Autodesk Inventor part; units mm, degrees
ref_plane "YZ Plane" through (0, 0, 0) normal (1, 0, 0) x (0, 1, 0)
ref_plane "XZ Plane" through (0, 0, 0) normal (0, 1, 0) x (-1, 0, 0)
ref_plane "XY Plane" through (0, 0, 0) normal (0, 0, 1) x (1, 0, 0)
sketch "Sketch1" plane through (0, 0, 0) normal (0, 0, 1) x (1, 0, 0)
  circle A0 centre (0, 0) radius 83.82
  dimension "d0" = 167.64
extrude "Extrusion1" add sketch "Sketch1" along normal mid plane 5.08
sketch "Sketch2" plane through (0, 0, 2.54) normal (0, 0, 1) x (1, 0, 0)
  circle A0 centre (0, 80.01) radius 1.7526
  circle A1 centre (-56.5756, 56.5756) radius 1.7526
  circle A2 centre (-80.01, 0) radius 1.7526
  circle A3 centre (-56.5756, -56.5756) radius 1.7526
  circle A4 centre (0, -80.01) radius 1.7526
  circle A5 centre (56.5756, -56.5756) radius 1.7526
  circle A6 centre (80.01, 0) radius 1.7526
  circle A7 centre (56.5756, 56.5756) radius 1.7526
  point P0 (0, 0)
  dimension "d3" = 3.5052
  dimension "d6" = 360
extrude "Extrusion2" cut sketch "Sketch2" against normal through all
sketch "Sketch3" plane through (0, 0, 2.54) normal (0, 0, 1) x (1, 0, 0)
  circle A0 centre (0, 40.9092) radius 1.7526
  circle A1 centre (-28.9272, 28.9272) radius 1.7526
  circle A2 centre (28.9272, 28.9272) radius 1.7526
  circle A3 centre (-40.9092, 0) radius 1.7526
  circle A4 centre (40.9092, 0) radius 1.7526
  circle A5 centre (0, -40.9092) radius 1.7526
  circle A6 centre (-28.9272, -28.9272) radius 1.7526
  circle A7 centre (28.9272, -28.9272) radius 1.7526
  point P0 (0, 0)
  point P1 (0, 0)
  point P2 (-37.0992, 0)
  dimension "d12" = 3.5052
  dimension "d16" = 45
  dimension "d20" = 45
  dimension "d24" = 45
  dimension "d28" = 45
extrude "Extrusion3" cut sketch "Sketch3" against normal through all
properties part number "EndCap"
The model under review builds one solid part; all positions refer to its coordinate system, in mm. Round coordinates to 2 decimals unless told otherwise and drop trailing zeros. Order: outer loops, then holes, each group sorted by start corner. A loop starts at its lowest first (then second) coordinate and runs counter-clockwise, first axis right, second up. Notation, with made-up numbers: (75, -39) - (98, -39) arc R16 ccw to (98, -16) - close; hole circle Ø1 at (-4, -11.5). An arc over 180 degrees is marked (long way). Answer in a Markdown table with one row per item.
(1) Take a section at A-A on z = -1.3. Count the separate pieces of the cut face and the enclosed holes in it, plus the area to 3 significant figures.
Result set:
| item | result |
|---|---|
| separate pieces | 1 |
| enclosed holes | 16 |
| area | 21,900 mm2 |
(2) For line 1 (Y direction, x = 0, z = -1.3); line 2 (Y direction, x = -58, z = 0.6); line 3 (X direction, y = 41.5, z = -1), list the stretches that pass through material, from the lowest coordinate up. Write a range as from..to.
Result set:
| item | result |
|---|---|
| line 1 | y = -83.82..-81.76, -78.26..-42.66, -39.16..39.16, 42.66..78.26, 81.76..83.82 |
| line 2 | y = -60.51..-57.6, -55.55..55.55, 57.6..60.51 |
| line 3 | x = -72.83..-1.65, 1.65..72.83 |
(3) Take a section at B-B on y = -50. Write out the cut boundary in (x, z), plus the area to 3 significant figures.
Result set:
| item | result |
|---|---|
| outline | (-67.27, -2.54) - (67.27, -2.54) - (67.27, 2.54) - (-67.27, 2.54) - close |
| area | 684 mm2 |
(4) Take a section at C-C on x = -22. Write out the cut boundary in (y, z).
Result set:
| item | result |
|---|---|
| outline | (-80.88, -2.54) - (80.88, -2.54) - (80.88, 2.54) - (-80.88, 2.54) - close |
(5) Clearance check with flat-ended pins moving along their axes: P1, Ø2, axis at x = -40.91, y = 0, coming from the +Z side; P2, Ø1.5, axis at y = 2.5, z = -2, coming from the +X side; P3, Ø4.5, axis at x = 0, y = 40.91, coming from the +Z side; P4, Ø1, axis at y = -11, z = 1, coming from the -X side. State where each tip first meets the part, or that it passes through.
Result set:
| item | result |
|---|---|
| P1 | passes through |
| P2 | stops at x = 83.8 |
| P3 | stops at z = 2.54 |
| P4 | stops at x = -83.16 |
